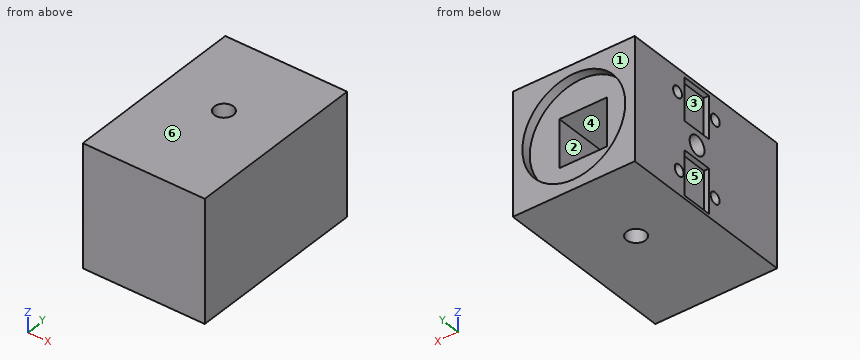
Autodesk Inventor part; units mm, degrees
ref_plane "YZ Plane" through (0, 0, 0) normal (1, 0, 0) x (0, 1, 0)
ref_plane "XZ Plane" through (0, 0, 0) normal (0, 1, 0) x (-1, 0, 0)
ref_plane "XY Plane" through (0, 0, 0) normal (0, 0, 1) x (1, 0, 0)
sketch "Sketch3" plane through (0, 0, 0) normal (0, 0, 1) x (1, 0, 0)
  line L0 (0, 0) -> (32, 0)
  line L1 (32, 0) -> (32, 48)
  line L2 (32, 48) -> (0, 48)
  line L3 (0, 48) -> (0, 0)
  dimension "d8" = 32
  dimension "d9" = 48
extrude "Extrusion2" add sketch "Sketch3" along normal blind 32
sketch "Sketch4" plane through (0, 48, 0) normal (0, 1, 0) x (1, 0, 0)
  line L0 (32, -32) -> (0, -32)
  line L1 (0, -32) -> (0, -16)
  line L2 (0, 0) -> (0, -32)
  line L3 (0, -16) -> (16, -16)
  circle A0 centre (16, -16) radius 13.5
  dimension "d12" = 16
  dimension "d13" = 16
  dimension "d14" = 27
sketch "Sketch5" plane through (0, 48, 0) normal (0, 1, 0) x (1, 0, 0)
  line L0 (15.9518, -16.0315) -> (15.9518, -9.2765)
  line L1 (15.9518, -9.2765) -> (9.1968, -9.2765)
  point P0 (0, 0)
  dimension "d15" = 6.755
  dimension "d16" = 6.755
sketch "Sketch6" plane through (0, 48, 0) normal (0, 1, 0) x (1, 0, 0)
  line L0 (9.1912, -9.2989) -> (9.1912, -21.8489)
  line L1 (9.1912, -21.8489) -> (21.7412, -21.8489)
  line L2 (21.7412, -21.8489) -> (21.7412, -9.2989)
  line L3 (21.7412, -9.2989) -> (9.1912, -9.2989)
  point P0 (0, 0)
  dimension "d17" = 12.55
  dimension "d18" = 12.55
  dimension "d19" = 12.55
  dimension "d20" = 12.55
extrude "Extrusion4" cut sketch "Sketch6" against normal blind 36
sketch "Sketch7" plane through (0, 0, 32) normal (0, 0, 1) x (1, 0, 0)
  line L0 (32, 48) -> (0, 48)
  line L1 (0, 48) -> (16, 48)
  line L2 (16, 48) -> (16, 27)
  circle A0 centre (16, 27) radius 2.5
  point P0 (0, 0)
  dimension "d25" = 16
  dimension "d26" = 21
  dimension "d27" = 5
hole "Hole1" at (16, 27, 32) direction (0, 0, -1) diameter 5 end through all
sketch "Sketch9" plane through (0, 0, 0) normal (-1, 0, 0) x (0, 0, 1)
  line L0 (0, 48) -> (16, 48)
  line L1 (21.8489, 48) -> (9.2989, 48)
  line L2 (16, 48) -> (16, 27)
  circle A0 centre (16, 27) radius 2.5
  point P0 (0, 0)
  dimension "d37" = 16
  dimension "d38" = 21
  dimension "d39" = 5
hole "Hole2" at (0, 27, 16) direction (1, 0, 0) diameter 5 depth 10 tip angle 118
sketch "Sketch10" plane through (21.7412, 48, 9.2989) normal (-1, 0, 0) x (0, 0, 1)
  circle A0 centre (6.7011, -21) radius 2.5
  line L0 (6.7011, -21) -> (6.7011, -9.86)
  line L1 (6.7011, -9.86) -> (6.7011, -21)
  line L2 (6.7011, -21) -> (6.7011, -9.86)
  line L3 (6.7011, -21) -> (6.7011, -32.14)
  line L4 (12.55, -36) -> (0, -36)
  line L5 (6.7011, -32.14) -> (6.7011, -21)
  line L6 (6.7011, -9.86) -> (21.6511, -9.86)
  line L7 (22.7011, -48) -> (22.7011, 0)
  line L8 (21.6511, -9.86) -> (6.7011, -9.86)
  line L9 (6.7011, -9.86) -> (-8.2489, -9.86)
  line L10 (21.6511, -9.86) -> (19.0973, -9.86)
  point P0 (-9.2989, -48)
  dimension "d47" = 11.14
  dimension "d48" = 11.14
  dimension "d49" = 14.95
  dimension "d50" = 14.95
sketch "Sketch11" plane through (0, 0, 0) normal (-1, 0, 0) x (0, 0, 1)
  line L0 (16.1419, 38.0227) -> (31.0919, 38.0227)
  line L1 (31.0919, 38.0227) -> (31.0919, 15.7427)
  line L2 (31.0919, 15.7427) -> (1.1919, 15.7427)
  line L3 (1.1919, 15.7427) -> (1.1919, 38.0227)
  line L4 (1.1919, 38.0227) -> (16.1419, 38.0227)
  line L5 (1.1919, 38.0227) -> (6.1919, 38.0227)
  line L6 (6.1919, 38.0227) -> (6.1919, 33.0227)
  circle A0 centre (6.1919, 33.0227) radius 1.7416
  point P0 (0, 0)
  dimension "d51" = 14.95
  dimension "d52" = 22.28
  dimension "d53" = 29.9
  dimension "d54" = 5
  dimension "d55" = 5
hole "Hole3" at (0, 33.0227, 6.1919) direction (1, 0, 0) diameter 3 depth 8 tip angle 118
sketch "Sketch12" plane through (0, 0, 0) normal (-1, 0, 0) x (0, 0, 1)
  point P0 (0, 0)
sketch "Sketch13" plane through (0, 0, 0) normal (-1, 0, 0) x (0, 0, 1)
  line L0 (30.9396, 38.5646) -> (25.9396, 38.5646)
  line L1 (25.9396, 38.5646) -> (25.9396, 33.5646)
  circle A0 centre (25.9396, 33.5646) radius 1.5
  point P0 (0, 0)
  dimension "d63" = 5
  dimension "d64" = 5
  dimension "d65" = 3
hole "Hole4" at (0, 33.5646, 25.9396) direction (1, 0, 0) diameter 3 depth 8 tip angle 118
sketch "Sketch14" plane through (0, 0, 0) normal (-1, 0, 0) x (0, 0, 1)
  line L0 (15.9777, 27.06) -> (1.0277, 27.06)
  line L1 (1.0277, 27.06) -> (1.0277, 15.92)
  line L2 (1.0277, 15.92) -> (6.0277, 15.92)
  line L3 (6.0277, 15.92) -> (6.0277, 20.92)
  circle A0 centre (6.0277, 20.92) radius 1.5
  point P0 (0, 0)
  dimension "d73" = 14.95
  dimension "d74" = 11.14
  dimension "d75" = 5
  dimension "d76" = 5
  dimension "d77" = 3
hole "Hole5" at (0, 20.92, 6.0277) direction (1, 0, 0) diameter 3 depth 8 tip angle 118
sketch "Sketch15" plane through (0, 0, 0) normal (-1, 0, 0) x (0, 0, 1)
  circle A0 centre (16, 27) radius 2.5
  line L0 (16, 27) -> (30.95, 27)
  line L1 (30.95, 27) -> (30.95, 15.86)
  line L2 (30.95, 15.86) -> (25.95, 15.86)
  line L3 (25.95, 15.86) -> (25.95, 20.86)
  circle A1 centre (25.95, 20.86) radius 1.5
  point P0 (0, 0)
  dimension "d85" = 14.95
  dimension "d86" = 11.14
  dimension "d87" = 5
  dimension "d88" = 5
  dimension "d89" = 3
hole "Hole6" at (0, 20.86, 25.95) direction (1, 0, 0) diameter 3 depth 8 tip angle 118
sketch "Sketch16" plane through (0, 0, 0) normal (-1, 0, 0) x (0, 0, 1)
  line L0 (0, 48) -> (0, 0)
  line L1 (0.7991, 31.1876) -> (12.4138, 31.1876)
  line L2 (9.2989, 48) -> (9.2989, 12)
  line L3 (12.4138, 31.1876) -> (12.4138, 22.9537)
  line L4 (12.4138, 22.9537) -> (0.7991, 22.9537)
  line L5 (0.7991, 22.9537) -> (0.7991, 31.1876)
extrude "Extrusion5" cut sketch "Sketch16" against normal blind 1.35
sketch "Sketch17" plane through (0, 0, 0) normal (-1, 0, 0) x (0, 0, 1)
  line L0 (19.8801, 31.1662) -> (30.9916, 31.1662)
  line L1 (30.9916, 31.1662) -> (30.9916, 23.0241)
  line L2 (30.9916, 23.0241) -> (19.8801, 23.0241)
  line L3 (19.8801, 23.0241) -> (19.8801, 31.1662)
  point P0 (0, 0)
extrude "Extrusion6" cut sketch "Sketch17" against normal blind 1.35
extrude "Extrusion7" cut sketch "Sketch4" against normal blind 2.5
properties part number "alan_optics_through_hole_chl_turbidity"
Here's how the part is built. I have some questions about the finished solid (model axes, mm). Face numbers are marked on the shaded views. A direction names the side the tool comes from. Give positions to 0.01 mm unless a question says otherwise; leave off trailing zeros. Loops run counter-clockwise (first coordinate to the right, second up) from the corner with the lowest first, then second, coordinate; pieces in that order, holes last. Notation, with made-up numbers: M -3,6 L 5,6 A28 cw 5,40 Z; hole C 53,81.25 d11. An arc over 180 degrees is marked long. Put each result on its own line as item: value. Start each with the question number.
(1) If we mould it in two halves opening along X, with no side actions, what happens to the marked faces 1, 2 and 3? For each: +X half, -X half, draft (parallel to the pull), parting line (faces both ways), or undercut.
(2) For the marked faces 4, 5 and 6, which set-ups out of +Z, -Z, +X, -X, +Y, -Y let a thin tool reach every point of the face, with its end or its side?
(3) I want a section at A-A on x = 16. Please give me the cut outline in (y, z).
(4) Will these pins go through, and if not, where does the flat tip stop? pin 1 Ø6 at (x, z) = (9, 11) entering from +Y; pin 2 Ø2.5 at (y, z) = (26, 26.5) entering from -X; pin 3 Ø10 at (x, z) = (16, 16.5) entering from +Y.
(5) I need wall thicknesses on line 1 along Z through (x, y) = (4.75, 20.92); line 2 along Y through (x, z) = (1.5, 25.95); line 3 along X through (y, z) = (38, 19). Which ranges of each line are inside material? Lowest first, please. Write a range as [from, to].
(6) I want a section at C-C on x = 25.5. Please give me the cut outline in (y, z), then the cut area to 3 significant figures.
(7) I want a section at B-B on x = 10.5. Please give me the cut outline in (y, z).
Answer block:
1. face 1: draft
1. face 2: undercut
1. face 3: -X half
2. face 4: +Y
2. face 5: -X
2. face 6: +Z, +X, -X, +Y, -Y
3. outline: M 0,0 L 24.5,0 L 24.5,9.3 L 12,9.3 L 12,21.85 L 24.5,21.85 L 24.5,32 L 0,32 Z; M 29.5,0 L 48,0 L 48,2.5 L 45.5,2.5 L 45.5,9.3 L 29.5,9.3 Z; M 29.5,21.85 L 45.5,21.85 L 45.5,29.5 L 48,29.5 L 48,32 L 29.5,32 Z
4. pin 1: y = 45.5
4. pin 2: x = 1.35
4. pin 3: y = 12
5. line 1: [0, 4.53], [7.53, 24.45], [27.45, 32]
5. line 2: [0, 19.36], [22.36, 32.06], [35.06, 48]
5. line 3: [0, 9.19], [21.74, 32]
6. outline: M 0,0 L 48,0 L 48,6.41 L 45.5,6.41 L 45.5,25.59 L 48,25.59 L 48,32 L 0,32 Z
6. area: 1,490 mm^2
7. outline: M 0,0 L 48,0 L 48,3.67 L 45.5,3.67 L 45.5,9.3 L 12,9.3 L 12,21.85 L 45.5,21.85 L 45.5,28.33 L 48,28.33 L 48,32 L 0,32 Z
